from build123d import *

# Parameters (mm, degrees)
F0_W = 58.8433295488
F0_H = 38.5233350098
F2_W = 13.3350025862
F2_H = 11.2183336169
F4_R = 5.08


with BuildPart() as f1:
    # F0 (on Front) → F1 (revolve)
    with BuildSketch(Plane.XZ):
        with Locations((29.4216647744, 19.2616675049)):
            Rectangle(F0_W, F0_H)
    revolve(axis=Axis((29.4216647744, 0, 0), (1, 0, 0)))

    # F2 (on Front) → F3 (revolve, cut)
    with BuildSketch(Plane.XZ):
        with Locations((28.2575013116, 35.8774987981)):
            Rectangle(F2_W, F2_H)
    revolve(axis=Axis((32.2791673243, 0, 0), (1, 0, 0)), mode=Mode.SUBTRACT)

    # F4
    f4_edges = [f1.edges().sort_by_distance(p)[0] for p in [
        (21.59, 0, -30.268332),
        (34.925003, 0, -30.268332),
        (28.257501, 0, 30.268332),
    ]]
    fillet(f4_edges, radius=F4_R)


solid = f1.part
Work out the finished part from the listing and answer in its coordinate system (mm). A direction names the side the tool comes from. Give positions to 0.01 mm unless a question says otherwise; leave off trailing zeros. Loops run counter-clockwise (first coordinate to the right, second up) from the corner with the lowest first, then second, coordinate; pieces in that order, holes last. Notation, with made-up numbers: (87, 61) - (128, 61) arc R22 cw to (128, 96) - close; hole circle Ø6 at (-1.75, 35.5). An arc over 180 degrees is marked (long way). Answer in a Markdown table with one row per item. Add a question column.
Q1. A tool of negligible diameter and unlimited length cuts with its end or side. For faces 1 (the flat face through (21.59, 16.94, -31.21)), 2 (the cylindrical face through (47.052, -11.571, 36.744)), from which of +Z, -Z, +X, -X, +Y, -Y can it reach the whole face along a straight path? Write none if from no direction.
Q2. Determine the mould class of faces 3 (the cylindrical face through (10.946, -11.571, 36.744)), 4 (the flat face through (58.843, -1, 1)), 5 (the flat face through (34.925, 16.94, -31.21)) for opening direction X: released by +X, released by -X, zero draft, split by the parting line, or undercut.
Q3. The part is cut by section C-C (x = 48). Determine the outline of the cut face in (y, z).
Q4. Consider line 1 along X through (y, z) = (-20, -30.5) (3 decimals); line 2 along X through (y, z) = (-10.5, 32); line 3 along Y through (x, z) = (18.5, -1). Determine where each line is inside the solid, lowest interval first.
Q5. The part is cut by section A-A (z = 0). Determine the outline of the cut face in (x, y) (3 decimals).
Q6. The part is cut by section D-D (x = 24.5). Determine the outline of the cut face in (y, z), and give its area (3 significant figures).
Q7. Each of these flat-tipped pins is pushed along its axis until it touches: P1, Ø12, axis at x = 49, y = -23.5, coming from the -Z side; P2, Ø6, axis at x = 41.5, y = -9.5, coming from the +Z side; P3, Ø4, axis at x = 7, z = -17, coming from the +Y side. Where does it stop, or does it pass through?
Solution:
| question | item | result |
|---|---|---|
| 1 | face 1 | none |
| 1 | face 2 | +X, -X |
| 2 | face 3 | zero draft |
| 2 | face 4 | released by +X |
| 2 | face 5 | undercut |
| 3 | outline | circle Ø77.05 at (0, 0) |
| 4 | line 1 | x = 0 to 21.59, 34.925 to 58.843 |
| 4 | line 2 | x = 0 to 21.87, 34.64 to 58.84 |
| 4 | line 3 | y = -38.51 to 38.51 |
| 5 | outline | (0, -38.523) - (21.59, -38.523) - (21.59, -35.348) arc R5.08 cw to (26.67, -30.268) - (29.845, -30.268) arc R5.08 cw to (34.925, -35.348) - (34.925, -38.523) - (58.843, -38.523) - (58.843, 38.523) - (34.925, 38.523) - (34.925, 35.348) arc R5.08 cw to (29.845, 30.268) - (26.67, 30.268) arc R5.08 cw to (21.59, 35.348) - (21.59, 38.523) - (0, 38.523) - close |
| 6 | outline | circle Ø61.51 at (0, 0) |
| 6 | area | 2,970 mm² |
| 7 | P1 | stops at z = -34.32 |
| 7 | P2 | stops at z = 37.97 |
| 7 | P3 | stops at y = 35.48 |
